from build123d import *

# Parameters (mm, degrees)
IZIM1_R                     = 7.75
Y_KSEKLIK_EKSTR_ZYON1_DEPTH = 4.5
IZIM2_R                     = 2.35
Y_KSEKLIK_EKSTR_ZYON2_DEPTH = 5
IZIM3_R                     = 3.1
KES_EKSTR_ZYON1_DEPTH       = 3.5


with BuildPart() as part:
    # Çizim1 → Yükseklik-Ekstrüzyon1 (new body)
    with BuildSketch(Plane(origin=(0, 0, 0), x_dir=(1, 0, 0), z_dir=(0, 1, 0))):
        Circle(IZIM1_R)
    extrude(amount=Y_KSEKLIK_EKSTR_ZYON1_DEPTH)

    # Çizim2 → Yükseklik-Ekstrüzyon2 (add)
    with BuildSketch(Plane(origin=(0, 4.5, 0), x_dir=(1, 0, 0), z_dir=(0, 1, 0))):
        Circle(IZIM2_R)
    extrude(amount=Y_KSEKLIK_EKSTR_ZYON2_DEPTH)

    # Çizim3 → Kes-Ekstrüzyon1 (cut)
    with BuildSketch(Plane.XZ):
        Circle(IZIM3_R)
    extrude(amount=-KES_EKSTR_ZYON1_DEPTH, mode=Mode.SUBTRACT)


solid = part.part
Here's how the part is built. I have some questions about the finished solid (model axes, mm). Give positions to 0.01 mm unless a question says otherwise; leave off trailing zeros. Loops run counter-clockwise (first coordinate to the right, second up) from the corner with the lowest first, then second, coordinate; pieces in that order, holes last. Notation, with made-up numbers: (89.5, 19) -> (105.5, 19) arc R16 ccw to (105.5, 37) -> close; hole circle Ø9 at (6, 3). An arc over 180 degrees is marked (long way). Answer as a JSON object with one key per item and string values. Group by question number.
Item 1: Imagine slicing it at C-C on z = 0. Write out the boundary of the cut face in (x, y).
Item 2: I need wall thicknesses on L1, parallel to Z at x = 0, y = 1.15; L2, parallel to Y at x = 0.75, z = 1; L3, parallel to Y at x = -0.75, z = -3.5. Which ranges of each line are inside material? Lowest first, please.
Item 3: Imagine slicing it at A-A on x = 0. Write out the boundary of the cut face in (y, z).
Item 4: Will these pins go through, and if not, where does the flat tip stop? pin 1 (4 mm diameter, centred on y = 4, z = -4.5, fed in from -X); pin 2 (5 mm diameter, centred on x = 5, y = 3.5, fed in from +Z); pin 3 (1 mm diameter, centred on y = 4, z = 4, fed in from +X); pin 4 (7 mm diameter, centred on x = 0, z = -1, fed in from -Y).
Item 5: Imagine slicing it at B-B on y = 2. Write out the boundary of the cut face in (x, z), then the cut area to 3 significant figures.
Item 6: Thinking about a two-plate mould opening in Z: for faces 1 (the cylindrical face through (1.43, 1.73, -2.75)), 2 (the cylindrical face through (-0.509, 6.965, 2.294)), 3 (the flat face through (0, 3.5, 0)), 4 (the flat face through (-2, 4.5, 2)), which applies, pulls with the +Z half, pulls with the -Z half, needs draft (parallel to the pull), parting line crosses it, or undercut?
Item 7: Imagine slicing it at D-D on y = 7.75. Write out the boundary of the cut face in (x, z).
Answer list:
{
 "1": {"outline": "(-7.75, 0) -> (-3.1, 0) -> (-3.1, 3.5) -> (3.1, 3.5) -> (3.1, 0) -> (7.75, 0) -> (7.75, 4.5) -> (2.35, 4.5) -> (2.35, 9.5) -> (-2.35, 9.5) -> (-2.35, 4.5) -> (-7.75, 4.5) -> close"},
 "2": {"L1": "z = -7.75 to -3.1, 3.1 to 7.75", "L2": "y = 3.5 to 9.5", "L3": "y = 0 to 4.5"},
 "3": {"outline": "(0, -7.75) -> (4.5, -7.75) -> (4.5, -2.35) -> (9.5, -2.35) -> (9.5, 2.35) -> (4.5, 2.35) -> (4.5, 7.75) -> (0, 7.75) -> (0, 3.1) -> (3.5, 3.1) -> (3.5, -3.1) -> (0, -3.1) -> close"},
 "4": {"pin 1": "stops at x = -7.34", "pin 2": "stops at z = 7.34", "pin 3": "stops at x = 6.91", "pin 4": "stops at y = 0"},
 "5": {"outline": "circle Ø15.5 at (0, 0); hole circle Ø6.2 at (0, 0)", "area": "159 mm2"},
 "6": {"face 1": "undercut", "face 2": "parting line crosses it", "face 3": "undercut", "face 4": "needs draft"},
 "7": {"outline": "circle Ø4.7 at (0, 0)"}
}
